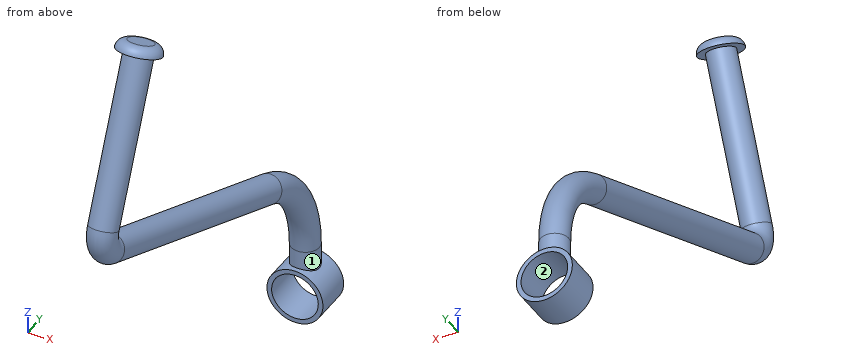
from build123d import *

# Parameters (mm, degrees)
SKETCH2_R                = 7.62
SKETCH4_R                = 11.950330427
BOSS_EXTRUDE1_DEPTH      = 5.08
FILLET1_R                = 5.08
BOSS_EXTRUDE2_DEPTH      = 10.16
BOSS_EXTRUDE2_DEPTH_BACK = 10.16
SKETCH5_R                = 15.24
SKETCH6_R                = 12.7
CUT_EXTRUDE1_DEPTH       = 335.141301153


with BuildPart() as part:
    # Sweep1: sweep along a path in Sketch1
    with BuildLine(Plane(origin=(0, 0, 0), x_dir=(0, 0, -1), z_dir=(1, 0, 0))) as sweep1_path:
        Line((-245.842907084, -163.312870299), (-164.080363385, -198.214108787))
        ThreePointArc((-164.080363385, -198.214108787), (-154.360765503, -198.318567045), (-147.414108787, -191.519636615))
        Line((-147.414108787, -191.519636615), (-81.467540759, -37.02772218))
        ThreePointArc((-81.467540759, -37.02772218), (-58.996512939, -10.092361683), (-25.401796509, 0))
        Line((-25.401796509, 0), (0, 0))
    # Sketch2 → Sweep1 (sweep)
    with BuildSketch(Plane.XY):
        Circle(SKETCH2_R)
    sweep(path=sweep1_path.line)

    # Sketch4 → Boss-Extrude1 (add)
    with BuildSketch(Plane(origin=(0, 63.595671041, 148.98450765), x_dir=(1, 0, 0), z_dir=(0, 0.39258985925704815, 0.9197136523986861))):
        with Locations(Location((0, -246.716508718, 0), (0, 0, 270))):
            Circle(SKETCH4_R)
    extrude(amount=BOSS_EXTRUDE1_DEPTH)

    # Fillet1
    fillet1_edges = [part.edges().sort_by_distance(p)[0] for p in [
        (0, -150.32763177, 245.823473898),
    ]]
    fillet(fillet1_edges, radius=FILLET1_R - 0.0001)  # a hair under: the kernel refuses the full size

    # Sketch5 → Boss-Extrude2 (add, two sides: drawn at the far end of the back side and taken through both)
    with BuildSketch(Plane(origin=(0, 0, 0), x_dir=(1, 0, 0), z_dir=(0, 1, 0)).offset(-BOSS_EXTRUDE2_DEPTH_BACK)):
        with Locations(Location((0, 0, 0), (0, 0, 270))):
            Circle(SKETCH5_R)
    extrude(amount=BOSS_EXTRUDE2_DEPTH + BOSS_EXTRUDE2_DEPTH_BACK)

    # Sketch6 → Cut-Extrude1 (cut, through all)
    with BuildSketch(Plane(origin=(0, 10.16, 0), x_dir=(1, 0, 0), z_dir=(0, 1, 0))):
        with Locations(Location((0, 0, 0), (0, 0, 270))):
            Circle(SKETCH6_R)
    extrude(amount=-CUT_EXTRUDE1_DEPTH, mode=Mode.SUBTRACT)


solid = part.part
Verification items for the finished model (mm, model axes). Face numbers are marked on the shaded views. A direction names the side the tool comes from. Round coordinates to 2 decimals unless told otherwise and drop trailing zeros. Order: outer loops, then holes, each group sorted by start corner. A loop starts at its lowest first (then second) coordinate and runs counter-clockwise, first axis right, second up.
1. Go/stop test with flat-tipped pins: P1, Ø5, axis at x = -2, y = -154, coming from the -Z side; P2, Ø3, axis at x = -1.5, y = -128, coming from the +Z side; P3, Ø2, axis at x = -6.5, y = -70.5, coming from the +Z side. Record where each tip stops, or that it passes through.
Final values:
P1: stops at z = 122.2
P2: stops at z = 129.12
P3: stops at z = 101.57
2. Access from +Z, -Z, +X, -X, +Y, -Y to the whole of each face (thin tool, end or side, straight path). Record for the marked faces 1 and 2.
Final values:
face 1: none
face 2: +Y, -Y
3. Thickness scan on L1, parallel to X at y = 2.5, z = 0; L2, parallel to Z at x = -5, y = -4.5; L3, parallel to Y at x = -13, z = 1.5. Record the ranges inside material, lowest first.
Final values:
L1: x = -15.24 to -12.7, 12.7 to 15.24
L2: z = -14.4 to -11.67, 11.67 to 60.93
L3: y = -10.16 to 10.16
4. Section check A-A on z = 0. Record the cut outline in (x, y), then the cut area to 3 significant figures.
Final values:
outline: (-15.24, -10.16) - (-12.7, -10.16) - (-12.7, 10.16) - (-15.24, 10.16) - close; (12.7, -10.16) - (15.24, -10.16) - (15.24, 10.16) - (12.7, 10.16) - close
area: 103 mm2
